Design review of the part built by this model. Coordinates are the model's own, in mm. Face numbers are marked on the shaded views. Give positions to 0.01 mm unless a question says otherwise; leave off trailing zeros. One line per item, written item: value. Start each with the question number.
```python
from build123d import *

# Parameters (mm, degrees)
SKETCH2_R           = 11.1125
BOSS_EXTRUDE1_DEPTH = 3.048
SKETCH3_R           = 10.16
CUT_EXTRUDE1_DEPTH  = 1.27
SKETCH4_R           = 3.81
CUT_EXTRUDE2_DEPTH  = 1.27
FILLET1_R           = 15.08


with BuildPart() as part:
    # Sketch2 → Boss-Extrude1 (new body)
    with BuildSketch(Plane(origin=(0, 0, 0), x_dir=(1, 0, 0), z_dir=(0, 1, 0))):
        with Locations(Location((0, 0, 0), (0, 0, 90))):
            Circle(SKETCH2_R)
    extrude(amount=BOSS_EXTRUDE1_DEPTH)

    # Sketch3 → Cut-Extrude1 (cut)
    with BuildSketch(Plane(origin=(0, 3.048, 0), x_dir=(1, 0, 0), z_dir=(0, 1, 0))):
        with Locations(Location((0, 0, 0), (0, 0, 270))):
            Circle(SKETCH3_R)
    extrude(amount=-CUT_EXTRUDE1_DEPTH, mode=Mode.SUBTRACT)

    # Sketch4 → Cut-Extrude2 (cut)
    with BuildSketch(Plane(origin=(0, 0, 0), x_dir=(-1, 0, 0), z_dir=(0, -1, 0))):
        with Locations(Location((0, 0, 0), (0, 0, 90))):
            Circle(SKETCH4_R)
    extrude(amount=-CUT_EXTRUDE2_DEPTH, mode=Mode.SUBTRACT)

    # Fillet1
    # the kernel refuses this fillet: 15.08 mm, written as the material it takes off along each edge
    with BuildSketch(Plane(origin=(0, 0, 0), x_dir=(0, 0, -1), z_dir=(-1, 0, 0))) as fillet1_piece_1:
        with BuildLine():
            CenterArc((9.867251852, -15.08), FILLET1_R, 90, 23.682902999)
            Line((3.81, -1.27), (3.81, 0))
            Line((3.81, 0), (9.867251852, 0))
        make_face()
    revolve(axis=Axis((0, 0, 0), (0, -1, 0)), mode=Mode.SUBTRACT)


solid = part.part
```
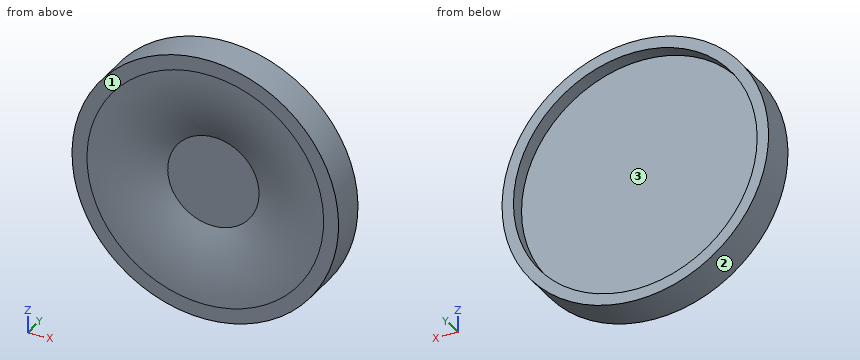
Q1. For P1, Ø2, axis at x = -4, z = 0, coming from the +Y side; P2, Ø12, axis at x = 0.5, z = -8.5, coming from the -Y side; P3, Ø8.5, axis at x = 1.5, z = -1.5, coming from the -Y side; P4, Ø1, axis at x = 1.5, y = 0.5, coming from the +Z side, all flat-tipped, find the tip position at first contact; note any pin that passes through.
Q2. Wall thickness on line 1 (X direction, y = 2.2, z = 0); line 2 (Z direction, x = -7, y = 2); line 3 (X direction, y = 2, z = -2.75): over which ranges is each line inside the solid? List them lowest first. Write a range as from..to.
Q3. The part is to be moulded in two halves that separate along X. For the marked faces 1, 2 and 3, say which applies: pulls with the +X half, pulls with the -X half, needs draft (parallel to the pull), parting line crosses it, or undercut.
Results list:
1. P1: stops at y = 1.78
1. P2: stops at y = 0
1. P3: stops at y = 0.41
1. P4: stops at z = 11.07
2. line 1: x = -11.11..-10.16, 10.16..11.11
2. line 2: z = -8.63..-7.36, 7.36..8.63
2. line 3: x = -10.77..-9.78, 9.78..10.77
3. face 1: needs draft
3. face 2: parting line crosses it
3. face 3: undercut
